Build history of the part. All positions in model axes, mm. A direction names the side the tool comes from. Round coordinates to 2 decimals unless told otherwise and drop trailing zeros. Write each loop counter-clockwise with the first axis right and the second up, starting at its lowest first coordinate (ties: lowest second). Pieces come first, ordered by that corner, then holes. Notation, with made-up numbers: (68, 7.5) - (111, 7.5) arc R21 ccw to (111, 27.5) - close; hole circle Ø6 at (-21.75, 69). An arc over 180 degrees is marked (long way). Write each question's results on one line, items separated by ' | '.
from build123d import *

# Parameters (mm, degrees)
F0_R      = 12.5
F1_DEPTH  = 175
F2_R      = 20
F3_DEPTH  = 10
F4_R      = 12.5
F5_DEPTH  = 10
F6_R      = 2.5
F7_R      = 2.5
F8_DEPTH  = 12.5
F9_R      = 1
F10_R     = 5
F11_SCALE = 0.24


with BuildPart() as f1:
    # F0 (on Right) → F1 (new body)
    with BuildSketch(Plane.YZ):
        Circle(F0_R)
    extrude(amount=F1_DEPTH)

    # F2 (on face) → F3 (join)
    with BuildSketch(Plane.YZ.offset(175)):
        Circle(F2_R)
    extrude(amount=F3_DEPTH)

    # F4 (on face) → F5 (join)
    with BuildSketch(Plane.YZ.offset(185)):
        Circle(F4_R)
    extrude(amount=F5_DEPTH)

    # F6
    f6_edges = [f1.edges().sort_by_distance(p)[0] for p in [
        (195, -12.5, 0),
        (185, -20, 0),
    ]]
    fillet(f6_edges, radius=F6_R)

    # F7 (on Front) → F8 (cut, symmetric)
    with BuildSketch(Plane.XZ):
        with Locations((22.5, 0)):
            Circle(F7_R)
    extrude(amount=F8_DEPTH, both=True, mode=Mode.SUBTRACT)

    # F9
    f9_edges = [f1.edges().sort_by_distance(p)[0] for p in [
        (22.5, 12.247449, 2.5),
        (22.5, 12.247449, -2.5),
        (20, -12.5, 0),
    ]]
    fillet(f9_edges, radius=F9_R)

    # F10
    f10_edges = [f1.edges().sort_by_distance(p)[0] for p in [
        (0, -12.5, 0),
    ]]
    fillet(f10_edges, radius=F10_R)


with BuildPart() as f1_1:
    # F11: moved
    add(f1.part.scale(F11_SCALE))


solid = f1_1.part
(1) Tool access for faces 4 (the flat face through (46.8, 0, 0)), 5 (the flat face through (44.4, -1, 3)), 6 (the cylindrical face through (21.31, 2.77, -1.15)): list every direction of +Z, -Z, +X, -X, +Y, -Y with a clear straight run to the whole face (end or side of a thin tool).
Worked answers:
face 4: +Z, -Z, +X, +Y, -Y | face 5: +X | face 6: -X
(2) Flat gauge pins, fed straight in: pin 1 Ø1.6 at (x, z) = (5.4, 0) entering from +Y; pin 2 Ø3 at (x, y) = (37, -1) entering from -Z; pin 3 Ø2 at (x, z) = (14.5, 3.5) entering from -Y. Where does each tip first touch, or does it go through?
Worked answers:
pin 1: stops at y = 3 | pin 2: stops at z = -3 | pin 3: stops at y = -1.66
(3) Drill centre lines: probe 1 along X at (y, z) = (1.65, 0); probe 2 along X at (y, z) = (-3.5, 0.25); probe 3 along Z at (x, y) = (5.4, 0.95). Where is each one in solid material? Low to high. Write a range as [from, to].
Worked answers:
probe 1: x = [0, 4.8], [6, 46.8] | probe 2: x = [42, 44.4] | probe 3: z = [-2.85, -0.6], [0.6, 2.85]
(4) Slice it at A-A, the plane y = 0. Write the cut outline in (x, z).
Worked answers:
outline: (0, -1.8) arc R1.2 ccw to (1.2, -3) - (42, -3) - (42, -4.8) - (43.8, -4.8) arc R0.6 ccw to (44.4, -4.2) - (44.4, -3) - (46.2, -3) arc R0.6 ccw to (46.8, -2.4) - (46.8, 2.4) arc R0.6 ccw to (46.2, 3) - (44.4, 3) - (44.4, 4.2) arc R0.6 ccw to (43.8, 4.8) - (42, 4.8) - (42, 3) - (1.2, 3) arc R1.2 ccw to (0, 1.8) - close; hole circle Ø1.2 at (5.4, 0)
(5) Two-plate mould, pull along Z, no slides. Class faces 1 (the flat face through (0, 0, 0)), 2 (the cylindrical face through (6, 0, 0)), 3 (the cylindrical face through (42.89, 2.58, 4.05)): released by +Z, released by -Z, zero draft, split by the parting line, or undercut.
Worked answers:
face 1: zero draft | face 2: undercut | face 3: split by the parting line
(6) Slice it at B-B, the plane x = 4. Write the cut outline in (y, z), and give its area (3 significant figures).
Worked answers:
outline: circle Ø6 at (0, 0) | area: 28.3 mm2
